Build history of the part. All positions in model axes, mm. Round coordinates to 2 decimals unless told otherwise and drop trailing zeros. Write each loop counter-clockwise with the first axis right and the second up, starting at its lowest first coordinate (ties: lowest second). Pieces come first, ordered by that corner, then holes. Notation, with made-up numbers: (-36.5, 78.5) -> (-2.5, 78.5) arc R19 cw to (-2.5, 85.5) -> close; hole circle Ø8 at (17, 70.25). An arc over 180 degrees is marked (long way). Answer in a Markdown table with one row per item.
```python
from build123d import *

# Parameters (mm, degrees)
F0_W        = 900
F0_H        = 150
F1_DEPTH    = 30
F2_T1_DEPTH = 1188.6630226256
F3_T1_DEPTH = 405.2304260538
F3_T3_DEPTH = 1086.1451046899


# Not quite as in the source:
# - a fillet or chamfer that OpenCascade refuses, or shapes differently, is made with other operations: its cross-section is extruded or revolved along the edge and cut away or added


with BuildPart() as f1:
    # F0 (on Front) → F1 (new body)
    with BuildSketch(Plane.XZ):
        with Locations((-450, -75)):
            Rectangle(F0_W, F0_H)
    extrude(amount=F1_DEPTH)

    # F2: fillet of radius 254 on 1 edges, made by hand

    # F2_s2 → F2_t1 (cut)
    with BuildSketch(Plane.XZ.offset(-579.3315113128)):
        with BuildLine():
            ThreePointArc((0, -150), (-93.7108671067, -40.7724220463), (-231.7326045251, 0))
            Line((-231.7326045251, 0), (0, 0))
            Line((0, 0), (0, -150))
        make_face()
    extrude(amount=F2_T1_DEPTH, mode=Mode.SUBTRACT)

    # F3: fillet of radius 38.1 on 2 edges, made by hand

    # F3_s2 → F3_t1 (cut)
    with BuildSketch(Plane.XZ.offset(-187.6152130269)):
        with BuildLine():
            ThreePointArc((-69.1890718946, -150), (-34.4974048158, -127.6511344129), (-40.5049190775, -86.8235294118))
            ThreePointArc((-40.5049190775, -86.8235294118), (-17.9063471748, -116.9075798319), (0, -150))
            Line((0, -150), (-69.1890718946, -150))
        make_face()
    extrude(amount=F3_T1_DEPTH, mode=Mode.SUBTRACT)

    # F3_s4 → F3_t3 (cut)
    with BuildSketch(Plane.YZ.offset(-993.0725523449)):
        with BuildLine():
            ThreePointArc((-30, -150), (-8.4333520599, -136.6770452378), (0, -112.770979062))
            Line((0, -112.770979062), (0, -150))
            Line((0, -150), (-30, -150))
        make_face()
    extrude(amount=F3_T3_DEPTH, mode=Mode.SUBTRACT)


solid = f1.part
```
Q1. Saw through at B-B on z = -19.5. Write the cut outline in (x, y), plus the area to 3 significant figures.
A:
| item | result |
|---|---|
| outline | (-900, -30) -> (-134.13, -30) -> (-134.13, 0) -> (-900, 0) -> close |
| area | 23,000 mm² |
Q2. Saw through at C-C on x = -261.5. Write the cut outline in (y, z).
A:
| item | result |
|---|---|
| outline | (-30, -150) arc R38.1 ccw to (0, -112.77) -> (0, 0) -> (-30, 0) -> close |
Q3. Drop flat-ended pins along their axis: P1, Ø3, axis at x = -744.5, y = -12, coming from the -Z side; P2, Ø8, axis at y = -13, z = -105, coming from the +X side; P3, Ø4, axis at x = -743, z = -17, coming from the +Y side; P4, Ø4, axis at x = -573.5, y = -22, coming from the -Z side. Give the stop position or say it passes through.
A:
| item | result |
|---|---|
| P1 | z = -141.86 |
| P2 | x = -31.2 |
| P3 | y = 0 |
| P4 | z = -148.17 |
Q4. Saw through at A-A on y = -10. Write the cut outline in (x, z).
A:
| item | result |
|---|---|
| outline | (-900, -138.5) -> (-41.91, -138.5) arc R38.1 ccw to (-40.5, -86.82) arc R254 ccw to (-231.73, 0) -> (-900, 0) -> close |
Q5. Wall check: line 1 (X direction, y = -15.5, z = -105.5); line 2 (X direction, y = -23.5, z = -54); line 3 (Z direction, x = -302.5, y = -12). Give the ranges that are in metal, low to high. Write a range as [from, to].
A:
| item | result |
|---|---|
| line 1 | [-900, -31.63] |
| line 2 | [-900, -75.16] |
| line 3 | [-140.53, 0] |
